from build123d import *

# Parameters (mm, degrees)
ESQUISSE1_W             = 100
ESQUISSE1_H             = 75
BOSS_EXTRU_1_DEPTH      = 47
COQUE1_T                = -6
ESQUISSE6_R             = 1.75
ENL_V_MAT_EXTRU_1_DEPTH = 7.3
ESQUISSE7_R             = 10
ENL_V_MAT_EXTRU_2_DEPTH = 0.5
ESQUISSE9_R             = 0.455
ESQUISSE9_R_2           = 1.6
ESQUISSE9_W             = 12
ESQUISSE9_H             = 7
ESQUISSE9_W_2           = 23.65
ENL_V_MAT_EXTRU_3_DEPTH = 6
ESQUISSE10_R            = 5.15
ENL_V_MAT_EXTRU_4_DEPTH = 6
ESQUISSE11_R            = 7.75
ENL_V_MAT_EXTRU_5_DEPTH = 3
CONG_1_R                = 2


with BuildPart() as part:
    # Esquisse1 → Boss.-Extru.1 (new body)
    with BuildSketch(Plane.XY):
        Rectangle(ESQUISSE1_W, ESQUISSE1_H)
    extrude(amount=BOSS_EXTRU_1_DEPTH)

    # Coque1
    coque1_openings = [part.faces().sort_by_distance(p)[0] for p in [
        (0, 0, 47),
    ]]
    offset(amount=COQUE1_T, openings=coque1_openings, kind=Kind.INTERSECTION)

    # Esquisse6 → Enlèv. mat.-Extru.1 (cut)
    with BuildSketch(Plane.XY.offset(47)):
        with Locations((-47, 34.5)):
            Circle(ESQUISSE6_R)
        with Locations(Location((47, 34.5, 0), (0, 0, 180))):
            Circle(ESQUISSE6_R)
        with Locations((47, -34.5)):
            Circle(ESQUISSE6_R)
        with Locations(Location((-47, -34.5, 0), (0, 0, 180))):
            Circle(ESQUISSE6_R)
    extrude(amount=-ENL_V_MAT_EXTRU_1_DEPTH, mode=Mode.SUBTRACT)

    # Esquisse7 → Enlèv. mat.-Extru.2 (cut)
    with BuildSketch(Plane(origin=(0, 0, 0), x_dir=(-1, 0, 0), z_dir=(0, 0, -1))):
        with Locations((-35, 22.5)):
            Circle(ESQUISSE7_R)
        with Locations(Location((35, 22.5, 0), (0, 0, 180))):
            Circle(ESQUISSE7_R)
        with Locations(Location((-35, -22.5, 0), (0, 0, 180))):
            Circle(ESQUISSE7_R)
        with Locations((35, -22.5)):
            Circle(ESQUISSE7_R)
    extrude(amount=-ENL_V_MAT_EXTRU_2_DEPTH, mode=Mode.SUBTRACT)

    # Esquisse9 → Enlèv. mat.-Extru.3 (cut)
    with BuildSketch(Plane(origin=(0, 37.5, 0), x_dir=(1, 0, 0), z_dir=(0, 1, 0))):
        with Locations(Location((-4.73, -31, 0), (0, 0, 270))):
            Circle(ESQUISSE9_R)
        with Locations(Location((-2.23, -31, 0), (0, 0, 270))):
            Circle(ESQUISSE9_R)
        with Locations(Location((10, -20.5, 0), (0, 0, 270))):
            Circle(ESQUISSE9_R_2)
        with Locations(Location((-20.96, -31, 0), (0, 0, 270))):
            Circle(ESQUISSE9_R)
        with Locations(Location((-23.46, -31, 0), (0, 0, 270))):
            Circle(ESQUISSE9_R)
        with Locations(Location((-25.96, -31, 0), (0, 0, 270))):
            Circle(ESQUISSE9_R)
        with Locations(Location((-37, -20.5, 0), (0, 0, 270))):
            Circle(ESQUISSE9_R_2)
        with Locations((-0.38, -20.3)):
            Rectangle(ESQUISSE9_W, ESQUISSE9_H)
        with Locations((-20.785, -20.3)):
            Rectangle(ESQUISSE9_W_2, ESQUISSE9_H)
    extrude(amount=-ENL_V_MAT_EXTRU_3_DEPTH, mode=Mode.SUBTRACT)

    # Esquisse10 → Enlèv. mat.-Extru.4 (cut)
    with BuildSketch(Plane(origin=(0, 37.5, 0), x_dir=(1, 0, 0), z_dir=(0, 1, 0))):
        with Locations(Location((30, -35, 0), (0, 0, 270))):
            Circle(ESQUISSE10_R)
    extrude(amount=-ENL_V_MAT_EXTRU_4_DEPTH, mode=Mode.SUBTRACT)

    # Esquisse11 → Enlèv. mat.-Extru.5 (cut)
    with BuildSketch(Plane.XZ.offset(-31.5)):
        with Locations(Location((30, 35, 0), (0, 0, 270))):
            Circle(ESQUISSE11_R)
    extrude(amount=-ENL_V_MAT_EXTRU_5_DEPTH, mode=Mode.SUBTRACT)

    # Congé1
    cong_1_edges = [part.edges().sort_by_distance(p)[0] for p in [
        (50, -37.5, 23.5),
        (-50, -37.5, 23.5),
        (-50, 37.5, 23.5),
        (50, 37.5, 23.5),
    ]]
    fillet(cong_1_edges, radius=CONG_1_R)


solid = part.part
Work out the finished part from the listing and answer in its coordinate system (mm). A direction names the side the tool comes from. Round coordinates to 2 decimals unless told otherwise and drop trailing zeros. Write each loop counter-clockwise with the first axis right and the second up, starting at its lowest first coordinate (ties: lowest second). Pieces come first, ordered by that corner, then holes. Notation, with made-up numbers: M 52.5,-28 L 81.5,-28 A28 cw 81.5,5 Z; hole C 28,-19.5 d7. An arc over 180 degrees is marked long. Use a Markdown table: item, result.
1) The part is cut by section C-C on y = 22.5. Give the vertices of the cut face in (x, z), plus the area to 3 significant figures.
Taken from the geometry:
| item | result |
|---|---|
| outline | M -50,0 L -45,0 L -45,0.5 L -25,0.5 L -25,0 L 25,0 L 25,0.5 L 45,0.5 L 45,0 L 50,0 L 50,47 L 44,47 L 44,6 L -44,6 L -44,47 L -50,47 Z |
| area | 1,070 mm2 |
2) Consider line 1 (X direction, y = 35.55, z = 20.5); line 2 (Y direction, x = -47, z = 41.25); line 3 (X direction, y = 1.5, z = 36.5). Determine where each line is inside the solid, lowest interval first. Write a range as [from, to].
Taken from the geometry:
| item | result |
|---|---|
| line 1 | x = [-50, -38.6], [-35.4, -32.61], [-8.96, -6.38], [5.62, 8.4], [11.6, 50] |
| line 2 | y = [-37.5, -36.25], [-32.75, 32.75], [36.25, 37.5] |
| line 3 | x = [-50, -44], [44, 50] |
3) The part is cut by section B-B on x = -0.5. Give the vertices of the cut face in (y, z), plus the area to 3 significant figures.
Taken from the geometry:
| item | result |
|---|---|
| outline | M -37.5,0 L 37.5,0 L 37.5,16.8 L 31.5,16.8 L 31.5,6 L -31.5,6 L -31.5,47 L -37.5,47 Z; M 31.5,23.8 L 37.5,23.8 L 37.5,47 L 31.5,47 Z |
| area | 900 mm2 |
4) The part is cut by section D-D on x = 39. Give the vertices of the cut face in (y, z).
Taken from the geometry:
| item | result |
|---|---|
| outline | M -37.5,0 L -31.67,0 L -31.67,0.5 L -13.33,0.5 L -13.33,0 L 13.33,0 L 13.33,0.5 L 31.67,0.5 L 31.67,0 L 37.5,0 L 37.5,47 L 31.5,47 L 31.5,6 L -31.5,6 L -31.5,47 L -37.5,47 Z |
5) Determine the mould class of faces 1 (the face through (-1, 1, 0)), 2 (the face through (5.62, 35, 20)), 3 (the face through (0, 35, 16.8)) for opening direction X: pulls with the +X half, pulls with the -X half, needs draft (parallel to the pull), parting line crosses it, or undercut.
Taken from the geometry:
| item | result |
|---|---|
| face 1 | needs draft |
| face 2 | undercut |
| face 3 | undercut |
6) The part is cut by section A-A on z = 15. Give the vertices of the cut face in (x, y), plus the area to 3 significant figures.
Taken from the geometry:
| item | result |
|---|---|
| outline | M -50,-35.5 A2 ccw -48,-37.5 L 48,-37.5 A2 ccw 50,-35.5 L 50,35.5 A2 ccw 48,37.5 L -48,37.5 A2 ccw -50,35.5 Z; hole M -44,-31.5 L 44,-31.5 L 44,31.5 L -44,31.5 Z |
| area | 1,950 mm2 |
7) Flat-ended cylindrical pins translate along their axes: pin 1 (2 mm diameter, centred on x = -8.5, y = -13, fed in from +Z); pin 2 (9.5 mm diameter, centred on x = 30, z = 35, fed in from +Y). Find the tip coordinate at first contact, or state that the pin passes through.
Taken from the geometry:
| item | result |
|---|---|
| pin 1 | stops at z = 6 |
| pin 2 | stops at y = -31.5 |
8) Which of the six approach directions +Z, -Z, +X, -X, +Y, -Y give full straight-line access (tool end or side, diameter ignored) to faces 4 (the face through (9.03, 34.54, 19.23)), 5 (the face through (-45.383, 33.83, 43.401)), 6 (the face through (35, 23, 0.5))?
Taken from the geometry:
| item | result |
|---|---|
| face 4 | +Y |
| face 5 | +Z |
| face 6 | -Z |
